Can you work these out from the model? Positions are in its coordinate system, mm. Give positions to 0.01 mm unless a question says otherwise; leave off trailing zeros. Loops run counter-clockwise (first coordinate to the right, second up) from the corner with the lowest first, then second, coordinate; pieces in that order, holes last. Notation, with made-up numbers: (-25.75, 23) - (19.25, 23) arc R24 ccw to (19.25, 37) - close; hole circle Ø1 at (64, 87.25). An arc over 180 degrees is marked (long way). Answer as a JSON object with one key per item and string values. Group by question number.
Item 1: Suppose I cut it at A-A on y = 3. Write out the boundary of the cut face in (x, z).
Item 2: Suppose I cut it at B-B on x = 18.5. Write out the boundary of the cut face in (y, z).
Item 3: Suppose I cut it at C-C on z = 1.45. Write out the boundary of the cut face in (x, y), and give its area (3 significant figures).
Item 4: Suppose I cut it at D-D on x = 6. Write out the boundary of the cut face in (y, z), and give its area (3 significant figures).
Item 5: Please list where these lines run through material, in increasing order: L1, parallel to X at y = 0.5, z = 1.55; L2, parallel to Y at x = -9, z = 3.5; L3, parallel to Y at x = 0, z = 3.
Item 6: Will this pin go through, and if not, where does the flat tip stop? pin 1 (1.5 mm diameter, centred on x = 6.5, z = 1.5, fed in from +Y).
Item 7: Thinking about a two-plate mould opening in Y: for faces 1 (the flat face through (5, 0, 5)), 2 (the cylindrical face through (1.32, 7.13, 2.46)), 3 (the cylindrical face through (16.9, -1.2, 2.5)), which applies, pulls with the +Y half, pulls with the -Y half, needs draft (parallel to the pull), parting line crosses it, or undercut?
from build123d import *

# Parameters (mm, degrees)
SKETCH1_R           = 1.25
SKETCH1_R_2         = 2
SKETCH1_R_3         = 0.75
BOSS_EXTRUDE1_DEPTH = 5


with BuildPart() as part:
    # Sketch1 → Boss-Extrude1 (new body)
    with BuildSketch(Plane.XY):
        with BuildLine():
            Line((-11.488369565, -0.131775361), (-4.510169836, -5.676342841))
            ThreePointArc((-4.510169836, -5.676342841), (-3.050109649, -6.577182613), (-1.419255622, -7.109726681))
            ThreePointArc((-1.419255622, -7.109726681), (9.701935293, -7.700842906), (20.533350493, -5.110331278))
            ThreePointArc((20.533350493, -5.110331278), (23.765864573, 1.587661896), (17.36972181, 5.382608217))
            ThreePointArc((17.36972181, 5.382608217), (9.957149012, 4.950641907), (2.743644121, 6.710805983))
            ThreePointArc((2.743644121, 6.710805983), (1.298650223, 7.132741941), (-0.202330164, 7.247176175))
            Line((-0.202330164, 7.247176175), (-9.111630435, 6.998442027))
            ThreePointArc((-9.111630435, 6.998442027), (-12.794733192, 4.264911064), (-11.488369565, -0.131775361))
        make_face()
        Circle(SKETCH1_R, mode=Mode.SUBTRACT)
        with Locations((18.5, 0)):
            Circle(SKETCH1_R_2, mode=Mode.SUBTRACT)
        with Locations((-9, 3)):
            Circle(SKETCH1_R_3, mode=Mode.SUBTRACT)
    extrude(amount=BOSS_EXTRUDE1_DEPTH)


solid = part.part
Worked out:
{
 "1": {"outline": "(-13, 0) - (-9.75, 0) - (-9.75, 5) - (-13, 5) - close; (-8.25, 0) - (23.11, 0) - (23.11, 5) - (-8.25, 5) - close"},
 "2": {"outline": "(-5.85, 0) - (-2, 0) - (-2, 5) - (-5.85, 5) - close; (2, 0) - (5.5, 0) - (5.5, 5) - (2, 5) - close"},
 "3": {"outline": "(-11.49, -0.13) - (-4.51, -5.68) arc R7.25 ccw to (-1.42, -7.11) arc R38.82 ccw to (20.53, -5.11) arc R5.5 ccw to (17.37, 5.38) arc R25.05 cw to (2.74, 6.71) arc R7.25 ccw to (-0.2, 7.25) - (-9.11, 7) arc R4 ccw to start; hole circle Ø1.5 at (-9, 3); hole circle Ø2.5 at (0, 0); hole circle Ø4 at (18.5, 0)", "area": "406 mm2"},
 "4": {"outline": "(-7.86, 0) - (5.63, 0) - (5.63, 5) - (-7.86, 5) - close", "area": "67.5 mm2"},
 "5": {"L1": "x = -12.12 to -1.15, 1.15 to 16.56, 20.44 to 23.98", "L2": "y = -2.11 to 2.25, 3.75 to 7", "L3": "y = -7.37 to -1.25, 1.25 to 7.25"},
 "6": {"pin 1": "stops at y = 5.7"},
 "7": {"face 1": "needs draft", "face 2": "pulls with the +Y half", "face 3": "undercut"}
}
